Build history of the part. All positions in model axes, mm. A direction names the side the tool comes from. Coordinates: 2 decimals unless noted, no trailing zeros. Loops run counter-clockwise (first coordinate to the right, second up) from the corner with the lowest first, then second, coordinate; pieces in that order, holes last. Notation, with made-up numbers: (58.5, -2) - (73.5, -2) arc R27 ccw to (73.5, 26) - close; hole circle Ø9 at (-10.75, 14). An arc over 180 degrees is marked (long way). One line per item, written item: value.
```python
from build123d import *

# Parameters (mm, degrees)
F1_DEPTH = 19.05
F2_R     = 11.43
F3_W     = 17.78
F3_H     = 12.7
F4_DEPTH = 25.4


with BuildPart() as f1:
    # F0 (on Front) → F1 (new body)
    with BuildSketch(Plane.XZ):
        with BuildLine():
            Line((0, 102.87), (0, 0))
            Line((0, 0), (214.63, 0))
            Line((214.63, 0), (214.63, 102.87))
            ThreePointArc((214.63, 102.87), (211.282230509, 110.952230509), (203.2, 114.3))
            Line((203.2, 114.3), (11.43, 114.3))
            ThreePointArc((11.43, 114.3), (3.347769491, 110.952230509), (0, 102.87))
        make_face()
    extrude(amount=F1_DEPTH)

    # F2
    f2_edges = [f1.edges().sort_by_distance(p)[0] for p in [
        (107.315, 0, 114.3),
    ]]
    fillet(f2_edges, radius=F2_R)

    # F3 (on face) → F4 (cut)
    with BuildSketch(Plane.XZ.offset(19.05)):
        with Locations((46.99, 19.05)):
            Rectangle(F3_W, F3_H)
    extrude(amount=-F4_DEPTH, mode=Mode.SUBTRACT)


solid = f1.part
```
Item 1: Probe probe 1 along X at (y, z) = (-11.5, 103.5); probe 2 along Y at (x, z) = (94, 103); probe 3 along Z at (x, y) = (142.5, -5.75). List the from-to ranges inside material, lowest first. Write a range as from..to.
Check result:
probe 1: x = 0.02..214.61
probe 2: y = -19.05..0
probe 3: z = 0..112.79
Item 2: Tool access for faces 1 (the face through (0, -15, 52)), 2 (the face through (55.88, -10, 19)): list every direction of +Z, -Z, +X, -X, +Y, -Y with a clear straight run to the whole face (end or side of a thin tool).
Check result:
face 1: +Z, -Z, -X, +Y, -Y
face 2: +Y, -Y
Item 3: Pull direction Z, two halves, no side cores. Call faces 3 (the face through (105.973, -3.437, 111.041)), 4 (the face through (3.259, -3.437, 50.715)), 5 (the face through (38.1, -10, 19)): released by +Z, released by -Z, zero draft, split by the parting line, or undercut.
Check result:
face 3: released by +Z
face 4: zero draft
face 5: undercut
Item 4: Drop flat-ended pins along their axis: P1, Ø1, axis at x = 76, y = -5, coming from the +Z side; P2, Ø4, axis at y = -6, z = 90.5, coming from the -X side; P3, Ø6.5, axis at y = -5.5, z = 22, coming from the -X side. Give the stop position or say it passes through.
Check result:
P1: stops at z = 112.64
P2: stops at x = 0.53
P3: stops at x = 0.32
Item 5: Cut at A-A, the plane y = -8.75. Write the cut outline in (x, z).
Check result:
outline: (0.32, 0) - (214.31, 0) - (214.31, 102.87) arc R11.11 ccw to (203.2, 113.98) - (11.43, 113.98) arc R11.11 ccw to (0.32, 102.87) - close; hole (38.1, 12.7) - (55.88, 12.7) - (55.88, 25.4) - (38.1, 25.4) - close
